from build123d import *

# Parameters (mm, degrees)
BOSS_EXTRUDE1_DEPTH = 100
CUT_EXTRUDE1_DEPTH  = 98
BOSS_EXTRUDE2_DEPTH = 240
CUT_EXTRUDE2_DEPTH  = 305


with BuildPart() as part:
    # Sketch1 → Boss-Extrude1 (new body)
    with BuildSketch(Plane.XY):
        with BuildLine():
            Line((-105, 181.865334795), (-100, 173.205080757))
            ThreePointArc((-100, 173.205080757), (0, 200), (100, 173.205080757))
            Line((100, 173.205080757), (105, 181.865334795))
            ThreePointArc((105, 181.865334795), (0, 210), (-105, 181.865334795))
        make_face()
    extrude(amount=BOSS_EXTRUDE1_DEPTH)

    # Sketch2 → Cut-Extrude1 (cut)
    with BuildSketch(Plane(origin=(0, 0, 1), x_dir=(-1, 0, 0), z_dir=(0, 0, -1))):
        with BuildLine():
            Line((99.632730807, 174.568951855), (103.632778417, 181.497237548))
            ThreePointArc((103.632778417, 181.497237548), (0, 209), (-103.632778417, 181.497237548))
            Line((-103.632778417, 181.497237548), (-99.632730807, 174.568951855))
            ThreePointArc((-99.632730807, 174.568951855), (0, 201), (99.632730807, 174.568951855))
        make_face()
        with BuildLine():
            Line((-104.132784113, 182.363272818), (-103.632778417, 181.497237548))
            ThreePointArc((-103.632778417, 181.497237548), (0, 209), (103.632778417, 181.497237548))
            Line((103.632778417, 181.497237548), (104.132784113, 182.363272818))
            ThreePointArc((104.132784113, 182.363272818), (0, 210), (-104.132784113, 182.363272818))
        make_face()
        with BuildLine():
            Line((-105.359240795, 184.487558104), (-104.132784113, 182.363272818))
            ThreePointArc((-104.132784113, 182.363272818), (0, 210), (104.132784113, 182.363272818))
            Line((104.132784113, 182.363272818), (105.359240795, 184.487558104))
            ThreePointArc((105.359240795, 184.487558104), (0, 213.475505009), (-105.359240795, 184.487558104))
        make_face()
    extrude(amount=-CUT_EXTRUDE1_DEPTH, mode=Mode.SUBTRACT)

    # Sketch3 → Boss-Extrude2 (add)
    with BuildSketch(Plane(origin=(0, 0, 0), x_dir=(1, 0, 0), z_dir=(0, 1, 0))):
        with BuildLine():
            ThreePointArc((-50.533623167, -30.054914333), (-69.052556755, -50), (-50.533623167, -69.945085667))
            ThreePointArc((-50.533623167, -69.945085667), (6.462857127, -69.523597841), (62.635134299, -59.856556138))
            ThreePointArc((62.635134299, -59.856556138), (70.947443245, -50), (62.635134299, -40.143443862))
            ThreePointArc((62.635134299, -40.143443862), (6.462857127, -30.476402159), (-50.533623167, -30.054914333))
        make_face()
    extrude(amount=BOSS_EXTRUDE2_DEPTH)

    # Sketch4 → Cut-Extrude2 (cut)
    with BuildSketch(Plane.XY):
        with BuildLine():
            Line((-69.052556755, 187.701210453), (-109.027774, 39.169052656))
            Line((-109.027774, 39.169052656), (-56.106611476, -33.467837082))
            Line((-56.106611476, -33.467837082), (100.062701462, -27.760652889))
            Line((100.062701462, -27.760652889), (70.947443245, 186.993209227))
            ThreePointArc((70.947443245, 186.993209227), (1.01141739, 199.997442571), (-69.052556755, 187.701210453))
        make_face()
    extrude(amount=CUT_EXTRUDE2_DEPTH, mode=Mode.SUBTRACT)


solid = part.part
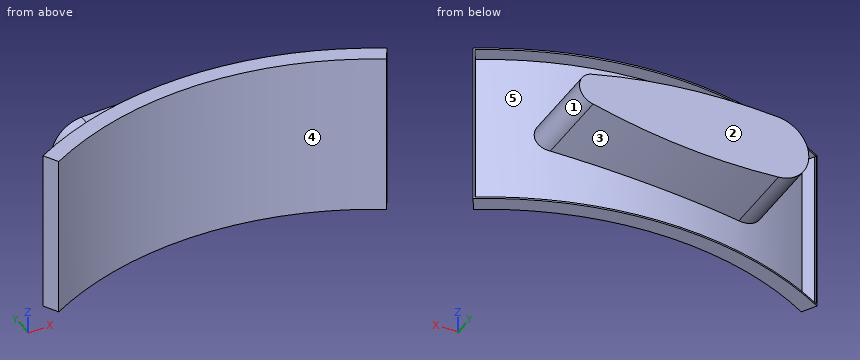
The model under review builds one solid part; all positions refer to its coordinate system, in mm. Face numbers are marked on the shaded views. A direction names the side the tool comes from. Coordinates: 2 decimals unless noted, no trailing zeros. Loops run counter-clockwise (first coordinate to the right, second up) from the corner with the lowest first, then second, coordinate; pieces in that order, holes last. Notation, with made-up numbers: (27.25, 67.25) -> (58.25, 67.25) arc R31 ccw to (58.25, 99.25) -> close; hole circle Ø6 at (-8.75, 63.5). An arc over 180 degrees is marked (long way). Use a Markdown table: item, result. Add a question column.
1. Add section D-D on x = 30.5. Write out the cut boundary in (y, z), plus the area to 3 significant figures.
2. Machinability: for the marked faces 4 and 5, which of the approach directions +Z, -Z, +X, -X, +Y, -Y give a long, thin tool a straight path to every point of the face, cutting with its end or side? Answer none if there is none.
3. Draft analysis for pull direction Z (two halves, no side actions). For the marked faces 1, 2 and 3, state which applies: pulls with the +Z half, pulls with the -Z half, needs draft (parallel to the pull), parting line crosses it, or undercut.
4. Add section A-A on y = 184.5. Write out the cut boundary in (x, z).
5. To check wall thickness, follow line 1 (X direction, y = 178, z = 66.5); line 2 (X direction, y = 180.5, z = 9.5) (3 decimals); line 3 (Y direction, x = 20.5, z = 50). State the ranges of each line that lie inside material, in increasing order.
6. Add section C-C on y = 206.5. Write out the cut boundary in (x, z), plus the area to 3 significant figures.
7. Add section B-B on z = 19. Write out the cut boundary in (x, y).
8. Clearance check with flat-ended pins moving along their axes: pin 1 Ø10 at (x, z) = (26, 62.5) entering from -Y; pin 2 Ø5 at (x, y) = (-31, 213.5) entering from -Z; pin 3 Ø1.5 at (y, z) = (203.5, 24.5) entering from -X; pin 4 Ø3 at (y, z) = (186, 90) entering from +X. State where each tip first meets the part, or that it passes through.
Returned:
| question | item | result |
|---|---|---|
| 1 | outline | (197.66, 0) -> (207.77, 0) -> (207.77, 1) -> (198.67, 1) -> (198.67, 33.46) -> (240, 33.46) -> (240, 66.54) -> (198.67, 66.54) -> (198.67, 99) -> (207.77, 99) -> (207.77, 100) -> (197.66, 100) -> close |
| 1 | area | 1,490 mm² |
| 2 | face 4 | +Z, -Z, -Y |
| 2 | face 5 | +Y |
| 3 | face 1 | undercut |
| 3 | face 2 | needs draft |
| 3 | face 3 | undercut |
| 4 | outline | (-100.3, 0) -> (-77.2, 0) -> (-77.2, 100) -> (-100.3, 100) -> (-100.3, 99) -> (-79.75, 99) -> (-79.75, 1) -> (-100.3, 1) -> close; (77.2, 0) -> (100.3, 0) -> (100.3, 1) -> (79.75, 1) -> (79.75, 99) -> (100.3, 99) -> (100.3, 100) -> (77.2, 100) -> close |
| 5 | line 1 | x = -102.77 to -101.61, -93.36 to -91.19, 91.19 to 93.36, 101.61 to 102.77 |
| 5 | line 2 | x = -104.212 to -103.057, -88.435 to -86.138, 86.138 to 88.435, 103.057 to 104.212 |
| 5 | line 3 | y = 198.95 to 240 |
| 6 | outline | (-50.53, 30.05) arc R350 ccw to (62.64, 40.14) arc R10 ccw to (62.64, 59.86) arc R350 ccw to (-50.53, 69.95) arc R20 ccw to start; (-38.18, 0) -> (38.18, 0) -> (38.18, 1) -> (-38.18, 1) -> close; (-38.18, 99) -> (38.18, 99) -> (38.18, 100) -> (-38.18, 100) -> close |
| 6 | area | 4,920 mm² |
| 7 | outline | (-105, 181.87) -> (-100, 173.21) arc R200 cw to (100, 173.21) -> (105, 181.87) arc R210 ccw to (104.13, 182.36) -> (99.63, 174.57) arc R201 ccw to (-99.63, 174.57) -> (-104.13, 182.36) arc R210 ccw to start |
| 8 | pin 1 | stops at y = 197.58 |
| 8 | pin 2 | stops at z = 29.12 |
| 8 | pin 3 | passes through |
| 8 | pin 4 | stops at x = 79.75 |
